Autodesk Inventor part; units mm, degrees
ref_plane "YZ Plane" through (0, 0, 0) normal (1, 0, 0) x (0, 1, 0)
ref_plane "XZ Plane" through (0, 0, 0) normal (0, 1, 0) x (-1, 0, 0)
ref_plane "XY Plane" through (0, 0, 0) normal (0, 0, 1) x (1, 0, 0)
sketch "Sketch1" plane through (0, 0, 0) normal (0, 1, 0) x (-1, 0, 0)
  line L0 (0, 0) -> (0, -14.74)
  arc A0 (-2.52, -14.74) -> (2.52, -14.74) centre (0, -14.74) ccw
  line L1 (2.4362, -15.3846) -> (4.3633, -0.5675)
  line L2 (-4.3633, -0.5675) -> (-2.4362, -15.3846)
  line L3 (0, 0) -> (0, 14.74)
  arc A1 (2.52, 14.74) -> (-2.52, 14.74) centre (0, 14.74) ccw
  circle A2 centre (0, 0) radius 4.4
  line L4 (2.4362, 15.3846) -> (4.3633, 0.5675)
  line L5 (-4.3633, 0.5675) -> (-2.4362, 15.3846)
  point P0 (4.3633, -0.5675)
  dimension "d2" = 2.52
extrude "Extrusion1" add sketch "Sketch1" along normal blind 2 contours L3 A2 L0 | L0 A2 L3 | A2 L1 A0 L2 | A2 L5 A1 L4
sketch "Sketch2" plane through (0, 2, 0) normal (0, 1, 0) x (1, 0, 0)
  circle A0 centre (0, 14.74) radius 0.7
  circle A1 centre (0, 12) radius 0.7
  circle A2 centre (0, 9.5) radius 0.7
  circle A3 centre (0, -14.74) radius 0.7
  circle A4 centre (0, -12) radius 0.7
  circle A5 centre (0, -9.5) radius 0.7
  point P0 (0, 0)
  dimension "d7" = 1.4
  dimension "d9" = 1.4
  dimension "d11" = 1.4
extrude "Extrusion2" cut sketch "Sketch2" against normal blind 2
sketch "Sketch3" plane through (0, 2, 0) normal (0, 1, 0) x (1, 0, 0)
  circle A0 centre (0, 0) radius 1.375
  dimension "d14" = 2.75
extrude "Extrusion3" cut sketch "Sketch3" against normal blind 2
sketch "Sketch4" plane through (0, 2, 0) normal (0, 1, 0) x (1, 0, 0)
  circle A0 centre (0, 0) radius 2.75
  circle A1 centre (0, 0) radius 3.785
  dimension "d18" = 5.5
  dimension "d19" = 7.57
extrude "Extrusion4" add sketch "Sketch4" along normal blind 0.45
sketch "Sketch5" plane through (0, 0, 0) normal (0, -1, 0) x (1, 0, 0)
  circle A0 centre (0, 0) radius 4.4
  dimension "d22" = 8.8
extrude "Extrusion5" add sketch "Sketch5" along normal blind 2
sketch "Sketch6" plane through (0, -2, 0) normal (0, -1, 0) x (1, 0, 0)
  circle A0 centre (0, 0) radius 1.375
  dimension "d25" = 2.75
extrude "Extrusion6" cut sketch "Sketch6" against normal blind 2
properties part number "MMAE 232 Assignment 2_White Propellor - Dylan Tamras"
Here's how the part is built. I have some questions about the finished solid (model axes, mm). A direction names the side the tool comes from. Coordinates: 2 decimals unless noted, no trailing zeros. Write each loop counter-clockwise with the first axis right and the second up, starting at its lowest first coordinate (ties: lowest second). Pieces come first, ordered by that corner, then holes.
1) Thinking about a two-plate mould opening in X: for faces 3 (the face through (0.05, 0.99, 17.26)), 4 (the face through (3.413, 0.986, 7.872)), 5 (the face through (-0.152, 1.014, 10.183)), 6 (the face through (3, 2.45, -1)), which applies, +X half, -X half, draft (parallel to the pull), parting line (faces both ways), or undercut?
Filled in:
face 3: parting line
face 4: +X half
face 5: undercut
face 6: draft
2) Which directions (+Z, -Z, +X, -X, +Y, -Y) give clear straight access to the entire face, cutting with the end or side of a thin tool? Please do faces 1 (the face through (-1.2, 2, -1.2)), 2 (the face through (2, -2, 0)).
Filled in:
face 1: +Y
face 2: +Z, -Z, +X, -X, -Y
3) I'm going to push flat-ended pins straight in: pin 1 (4.5 mm diameter, centred on x = 0, z = 0, fed in from +Y); pin 2 (5 mm diameter, centred on x = -3, z = -12.5, fed in from -Y); pin 3 (1 mm diameter, centred on y = 2, z = 4, fed in from -X). Where does each tip first touch, or does it pass through?
Filled in:
pin 1: stops at y = 2
pin 2: stops at y = 0
pin 3: stops at x = -3.98
4) If I drill on line 1 (Y direction, x = -0.75, z = 16); line 2 (X direction, y = 0.6, z = 12); line 3 (X direction, y = 1.3, z = 14.74), over which ranges is the centre line in solid material (lowest first)?
Filled in:
line 1: y = 0 to 2
line 2: x = -2.88 to -0.7, 0.7 to 2.88
line 3: x = -2.52 to -0.7, 0.7 to 2.52
5) If we section it at B-B (y = -1.3): List the corners of the cut face in (x, z) for me (3 decimals).
Filled in:
outline: circle Ø8.8 at (0, 0); hole circle Ø2.75 at (0, 0)
6) If we section it at A-A (z = -9.5): List the corners of the cut face in (x, y) for me.
Filled in:
outline: (-3.2, 0) - (-0.7, 0) - (-0.7, 2) - (-3.2, 2) - close; (0.7, 0) - (3.2, 0) - (3.2, 2) - (0.7, 2) - close
7) If we section it at C-C (x = 0): Count the separate pieces of the cut face and the enclosed holes in it, plus the area to 3 significant figures.
Filled in:
separate pieces: 8
enclosed holes: 0
area: 59.8 mm2
